Autodesk Inventor part; units mm, degrees
ref_plane "YZ Plane" through (0, 0, 0) normal (1, 0, 0) x (0, 1, 0)
ref_plane "XZ Plane" through (0, 0, 0) normal (0, 1, 0) x (-1, 0, 0)
ref_plane "XY Plane" through (0, 0, 0) normal (0, 0, 1) x (1, 0, 0)
sketch "スケッチ1" plane through (0, 0, 0) normal (0, 0, 1) x (1, 0, 0)
  line L0 (-17, -61.25) -> (17, -61.25) construction
  line L1 (17, -61.25) -> (17, 61.25) construction
  line L2 (17, 61.25) -> (-17, 61.25) construction
  line L3 (-17, 61.25) -> (-17, -61.25) construction
  line L4 (-17, -61.25) -> (17, 61.25) construction
  line L5 (17, -61.25) -> (-17, 61.25) construction
  line L6 (-17, 43.35) -> (-17, 61.25)
  line L7 (-17, 61.25) -> (17, 61.25)
  line L8 (17, 61.25) -> (17, 43.35)
  line L9 (-17, -43.35) -> (-17, -61.25)
  line L10 (-17, -61.25) -> (17, -61.25)
  line L11 (17, -61.25) -> (17, -43.35)
  line L12 (-17, 41.25) -> (-22, 41.25)
  line L13 (-22, 41.25) -> (-22, -41.25)
  line L14 (-22, -41.25) -> (-17, -41.25)
  line L15 (17, 41.25) -> (22, 41.25)
  line L16 (22, 41.25) -> (22, -41.25)
  line L17 (22, -41.25) -> (17, -41.25)
  arc A0 (-17, 41.25) -> (-17, 43.35) centre (-17, 42.3) ccw
  arc A1 (-17, -43.35) -> (-17, -41.25) centre (-17, -42.3) ccw
  arc A2 (17, 43.35) -> (17, 41.25) centre (17, 42.3) ccw
  arc A3 (17, -41.25) -> (17, -43.35) centre (17, -42.3) ccw
  line L18 (0, 0) -> (17, 0) construction
  line L19 (0, 0) -> (0, 61.25) construction
  line L20 (-9.5, 56.25) -> (9.5, 56.25) construction
  line L21 (9.5, 56.25) -> (9.5, -5.75) construction
  line L22 (9.5, -5.75) -> (-9.5, -5.75) construction
  line L23 (-9.5, -5.75) -> (-9.5, 56.25) construction
  circle A4 centre (-9.5, 56.25) radius 1.6
  circle A5 centre (-9.5, -5.75) radius 1.6
  point P0 (0, 56.25)
  point P1 (0, 0)
  dimension "d87" = 1.05
  dimension "d88" = 122.5
  dimension "d89" = 5
  dimension "d90" = 20
  dimension "d91" = 34
  dimension "d92" = 3.2
  dimension "d93" = 7.5
  dimension "d94" = 5
  dimension "d112" = 62
extrude "押し出し1" add sketch "スケッチ1" along normal blind 5
sketch "スケッチ2" plane through (0, 0, 5) normal (0, 0, 1) x (1, 0, 0)
  line L0 (-17, 61.25) -> (-17, 43.35)
  line L1 (17, 43.35) -> (17, 61.25)
  line L2 (-40.5884, 60.19) -> (-17, 60.19)
  line L3 (-17, 60.19) -> (-17, -101.7483)
  line L4 (-17, -101.7483) -> (-40.5884, -101.7483)
  line L5 (-40.5884, -101.7483) -> (-40.5884, 60.19)
  line L6 (53.5752, 90.4043) -> (17, 90.4043)
  line L7 (17, 90.4043) -> (17, -93.5321)
  line L8 (17, -93.5321) -> (53.5752, -93.5321)
  line L9 (53.5752, -93.5321) -> (53.5752, 90.4043)
  point P0 (0, 0)
extrude "押し出し2" cut sketch "スケッチ2" against normal blind 2.5
sketch "スケッチ3" plane through (0, 0, 5) normal (0, 0, 1) x (1, 0, 0)
  line L0 (17, -41.25) -> (17, 41.25)
  line L1 (17, 61.25) -> (-17, 61.25)
  line L2 (-17, 41.25) -> (-17, -41.25)
  line L3 (-17, -61.25) -> (17, -61.25)
  circle A0 centre (-9.5, -5.75) radius 1.6
  circle A1 centre (-9.5, 56.25) radius 1.6
  line L4 (-7, -57.25) -> (7, -57.25)
  line L5 (7, -57.25) -> (7, -10.75)
  line L6 (7, -10.75) -> (-7, -10.75)
  line L7 (-7, -10.75) -> (-7, -57.25)
  line L8 (-12, 0.25) -> (12, 0.25)
  line L9 (12, 0.25) -> (12, 50.25)
  line L10 (12, 50.25) -> (-12, 50.25)
  line L11 (-12, 50.25) -> (-12, 0.25)
  line L12 (0, 61.25) -> (0, -61.25) construction
  line L13 (-17, 0) -> (17, 0) construction
  point P0 (0, 0)
  point P1 (0, 0.25)
  dimension "d100" = 4
  dimension "d105" = 11
  dimension "d108" = 5
  dimension "d114" = 6
  dimension "d115" = 10
  dimension "d116" = 6
extrude "押し出し3" cut sketch "スケッチ3" against normal blind 10 contours L7 L6 L5 L4 | L11 L10 L9 L8
fillet "フィレット1" radius 5 8 edges at (-7, -57.25, 2.5) (-7, -10.75, 2.5) (7, -57.25, 2.5) (7, -10.75, 2.5) (-12, 0.25, 2.5) (-12, 50.25, 2.5) (12, 0.25, 2.5) (12, 50.25, 2.5)
sketch "スケッチ5" plane through (0, 0, 5) normal (0, 0, 1) x (1, 0, 0)
  circle A0 centre (-9.5, 56.25) radius 1.6
  circle A1 centre (-9.5, -5.75) radius 1.6
  circle A2 centre (-9.5, -5.75) radius 3
  circle A3 centre (-9.5, 56.25) radius 3
  point P0 (0, 0)
  dimension "d117" = 6
  dimension "d118" = 6
extrude "押し出し4" cut sketch "スケッチ5" against normal blind 3.2
sketch "スケッチ7" plane through (-17, -61.25, 0) normal (-1, 0, 0) x (0, 0, 1)
  line L0 (0, 0) -> (0, 17.9)
  line L1 (5, 17.9) -> (5, 0)
  line L2 (0, 0) -> (5, 0)
  point P0 (0, 61.25)
  point P1 (2.5, 7.5)
  dimension "d130" = 5
  dimension "d131" = 7.5
  dimension "d132" = 2.5
hole "穴1" at (-17, -53.75, 2.5) direction (1, 0, 0) diameter 2.459 depth 12
sketch "スケッチ8" plane through (17, -61.25, 0) normal (1, 0, 0) x (0, 0, -1)
  line L0 (0, 0) -> (-5, 0)
  line L1 (-5, 0) -> (-5, 17.9)
  point P0 (0, 61.25)
  point P1 (-2.5, 7.5)
  dimension "d140" = 7.5
  dimension "d141" = 2.5
hole "穴2" at (17, -53.75, 2.5) direction (-1, 0, 0) diameter 2.459 depth 12
equation "\"d88\" = d83"
equation "\"d90\" = d84"
properties part number "コックピット_2_サブフレーム_5" material "アセタール樹脂、黒"
Design review of the part built by this model. Coordinates are the model's own, in mm. A direction names the side the tool comes from. Give positions to 0.01 mm unless a question says otherwise; leave off trailing zeros. Loops run counter-clockwise (first coordinate to the right, second up) from the corner with the lowest first, then second, coordinate; pieces in that order, holes last. Notation, with made-up numbers: M 34.5,27.5 L 40.5,27.5 A9 ccw 40.5,44.5 Z; hole C -38,-15.75 d1. An arc over 180 degrees is marked long. Write item = value, one per line.
Q1. We need section B-B (x = -9.5). Give the boundary of the cut face in (y, z).
Output values:
outline = M -61.25,0 L -7.35,0 L -7.35,1.8 L -8.75,1.8 L -8.75,5 L -61.25,5 Z; M -4.15,0 L 0.92,0 L 0.92,5 L -2.75,5 L -2.75,1.8 L -4.15,1.8 Z; M 49.58,0 L 54.65,0 L 54.65,1.8 L 53.25,1.8 L 53.25,5 L 49.58,5 Z; M 57.85,0 L 61.25,0 L 61.25,5 L 59.25,5 L 59.25,1.8 L 57.85,1.8 Z; hole C -53.75,2.5 d2.46
Q2. To check wall thickness, follow line 1 (Y direction, x = 2, z = 3.5); line 2 (X direction, y = 37, z = 0.95); line 3 (X direction, y = -49, z = 1.85). State the ranges of each line that lie inside material, in increasing order. Write a range as [from, to].
Output values:
line_1 = [-61.25, -57.25], [-10.75, 0.25], [50.25, 61.25]
line_2 = [-22, -12], [12, 22]
line_3 = [-17, -7], [7, 17]
Q3. Draft analysis for pull direction X (two halves, no side actions). For faces 1 (the cylindrical face through (11.52, -54.97, 2.66)), 2 (the cylindrical face through (-9.891, 59.224, 3.422)), 3 (the flat face through (-17, -52, 2)), 4 (the flat face through (17, -52, 2)), state which applies: +X half, -X half, draft (parallel to the pull), parting line (faces both ways), or undercut.
Output values:
face_1 = draft
face_2 = undercut
face_3 = -X half
face_4 = +X half
Q4. We need section A-A (y = -39.5). Give the boundary of the cut face in (x, z).
Output values:
outline = M -22,0 L -7,0 L -7,5 L -17,5 L -17,2.5 L -22,2.5 Z; M 7,0 L 22,0 L 22,2.5 L 17,2.5 L 17,5 L 7,5 Z
Q5. Insertion check: pin 1 (1.5 mm diameter, centred on y = -51, z = 3.5, fed in from +X); pin 2 (2.5 mm diameter, centred on y = 50.5, z = 3, fed in from -X). Each pin has a flat end and moves straight along its axis. Give the tip position at first contact, or say it passes through.
Output values:
pin_1 = 17
pin_2 = -17
Q6. We need section C-C (y = 56.25). Give the boundary of the cut face in (x, z).
Output values:
outline = M -17,0 L -11.1,0 L -11.1,1.8 L -12.5,1.8 L -12.5,5 L -17,5 Z; M -7.9,0 L 17,0 L 17,5 L -6.5,5 L -6.5,1.8 L -7.9,1.8 Z
Q7. We need section D-D (y = -1). Give the boundary of the cut face in (x, z).
Output values:
outline = M -22,0 L 22,0 L 22,2.5 L 17,2.5 L 17,5 L -17,5 L -17,2.5 L -22,2.5 Z
Q8. For faces 5 (the flat face through (-19, 41.25, 1)), 6 (the flat face through (19, 1, 2.5)), 7 (the cylindrical face through (10.57, 1.75, 2.46)), 8 (the flat face through (20, -41.25, 1)), list the 3-axis set-ups (+Z, -Z, +X, -X, +Y, -Y) from which the entire face can be reached by the end or side of a thin tool; tool diameter is ignored.
Output values:
face_5 = +Z, -Z, -X, +Y
face_6 = +Z, +X, +Y, -Y
face_7 = +Z, -Z
face_8 = +Z, -Z, +X, -Y
